```python
from build123d import *

# Parameters (mm, degrees)
SKETCH2_W           = 110
SKETCH2_H           = 8
BOSS_EXTRUDE1_DEPTH = 12
LPATTERN1_COUNT     = 5
LPATTERN1_PITCH     = 22
SKETCH4_R           = 2.05
CUT_EXTRUDE1_DEPTH  = 5
CUT_EXTRUDE1_TAPER  = 1


with BuildPart() as part:
    # Sketch2 → Boss-Extrude1 (new body)
    with BuildSketch(Plane.XY):
        with Locations((55, 4)):
            Rectangle(SKETCH2_W, SKETCH2_H)
    extrude(amount=-BOSS_EXTRUDE1_DEPTH)

    # Sketch3 → Cut-Revolve1 (revolve, cut)
    with BuildSketch(Plane.XY):
        Polygon((8, 3), (8.9, 3), (8.9, 5), (2, 5), (2, 6), (11, 6), (11, 0), (8.9, 0), align=None)
    cut_revolve1 = revolve(axis=Axis((11, 6, 0), (0, -1, 0)), mode=Mode.SUBTRACT)

    # LPattern1: Cut-Revolve1 ×5
    with Locations(*[(i * LPATTERN1_PITCH, 0, 0) for i in range(1, LPATTERN1_COUNT)]):
        add(cut_revolve1, mode=Mode.SUBTRACT)

    # Sketch4 → Cut-Extrude1 (cut)
    with BuildSketch(Plane.XY):
        with Locations((22, 3)):
            Circle(SKETCH4_R)
        with Locations((88, 3)):
            Circle(SKETCH4_R)
    extrude(amount=-CUT_EXTRUDE1_DEPTH, taper=CUT_EXTRUDE1_TAPER, mode=Mode.SUBTRACT)


solid = part.part
```
For this review, take the finished solid that the model builds, in its own axes (mm). A direction names the side the tool comes from. Coordinates: 2 decimals unless noted, no trailing zeros. Write each loop counter-clockwise with the first axis right and the second up, starting at its lowest first coordinate (ties: lowest second). Pieces come first, ordered by that corner, then holes. Notation, with made-up numbers: (5.25, 58.25) - (39.25, 58.25) arc R17 cw to (39.25, 90.25) - close; hole circle Ø3 at (54.5, -31.5). An arc over 180 degrees is marked (long way). Put each result on its own line as item: value.
1. Mouldability with a two-part tool opening along X and no side actions: class faces 4 (the flat face through (54, 7, 0)), 5 (the flat face through (0, 4, -6)), 6 (the cylindrical face through (77, 4, -2.1)) as released by +X, released by -X, zero draft, split by the parting line, or undercut.
Values found:
face 4: zero draft
face 5: released by -X
face 6: undercut
2. Wall thickness on probe 1 along Y at (x, z) = (25.5, -0.75); probe 2 along X at (y, z) = (5.25, -5.5); probe 3 along Z at (x, y) = (57, 5.25): over which ranges is each line inside the solid? List them lowest first.
Values found:
probe 1: 0 to 5, 6 to 8
probe 2: 0 to 3.88, 18.12 to 25.88, 40.12 to 47.88, 62.12 to 69.88, 84.12 to 91.88, 106.12 to 110
probe 3: -12 to -8.77
3. Machinability: for faces 1 (the flat face through (54, 0, -6)), 2 (the cylindrical face through (55, 4, -2.1)), 3 (the flat face through (55, 5, -4)), which of the approach directions +Z, -Z, +X, -X, +Y, -Y give a long, thin tool a straight path to every point of the face, cutting with its end or side? Answer none if there is none.
Values found:
face 1: +Z, -Z, +X, -X, -Y
face 2: +Z, -Y
face 3: +Z
4. Add section B-B, the plane z = -6.5. Give the boundary of the cut face in (x, y), then the cut area to 3 significant figures.
Values found:
outline: (0, 0) - (110, 0) - (110, 8) - (0, 8) - close; hole (4.78, 5) - (17.22, 5) - (17.22, 6) - (4.78, 6) - close; hole (26.78, 5) - (39.22, 5) - (39.22, 6) - (26.78, 6) - close; hole (48.78, 5) - (61.22, 5) - (61.22, 6) - (48.78, 6) - close; hole (70.78, 5) - (83.22, 5) - (83.22, 6) - (70.78, 6) - close; hole (92.78, 5) - (105.22, 5) - (105.22, 6) - (92.78, 6) - close
area: 818 mm²
5. Add section C-C, the plane z = -1. Count the separate pieces of the cut face and the enclosed holes in it, then the cut area to 3 significant figures.
Values found:
separate pieces: 1
enclosed holes: 2
area: 657 mm²
6. Add section A-A, the plane x = 33. Give the boundary of the cut face in (y, z).
Values found:
outline: (0, -12) - (8, -12) - (8, 0) - (6, 0) - (6, -9) - (5, -9) - (5, -2.1) - (3, -2.1) - (3, -3) - (0, -2.1) - close
7. For pin 1 (1.2 mm diameter, centred on x = 22.5, y = 3, fed in from +Z), flat-tipped, find the tip position at first contact; note if it passes through.
Values found:
pin 1: z = -5
